Answer from the drawing. Dimensions are ordinates in mm from the lowest x, y and z of the part. Round coordinates to 2 decimals unless told otherwise and drop trailing zeros. Order: outer loops, then holes, each group sorted by start corner. A loop starts at its lowest first (then second) coordinate and runs counter-clockwise, first axis right, second up. Notation, with made-up numbers: (28.25, 81) -> (54.25, 81) arc R31 cw to (54.25, 111) -> close; hole circle Ø5 at (49.5, 19). An arc over 180 degrees is marked (long way). Use a Markdown table: item, result. Add a question column.
1. Section A-A, the plane x = 22 is taken. Give the vertices of the cut face in (y, z), then the cut area to 3 significant figures.
2. The mould has two halves that part along Z. Classify the marked faces 1, 2 and 3: +Z half, -Z half, draft (parallel to the pull), parting line (faces both ways), or undercut.
3. Section B-B, the plane z = 26 is taken. Give the vertices of the cut face in (x, y).
4. Section C-C, the plane y = 37 is taken. Give the vertices of the cut face in (x, z) (1 decimal).
5. Consider L1, parallel to X at y = 6.5, z = 20.5; L2, parallel to Z at x = 31, y = 12.5 (1 decimal); L3, parallel to Z at x = 26, y = 30. Determine where each line is inside the solid, lowest interval first. Write a range as [from, to].
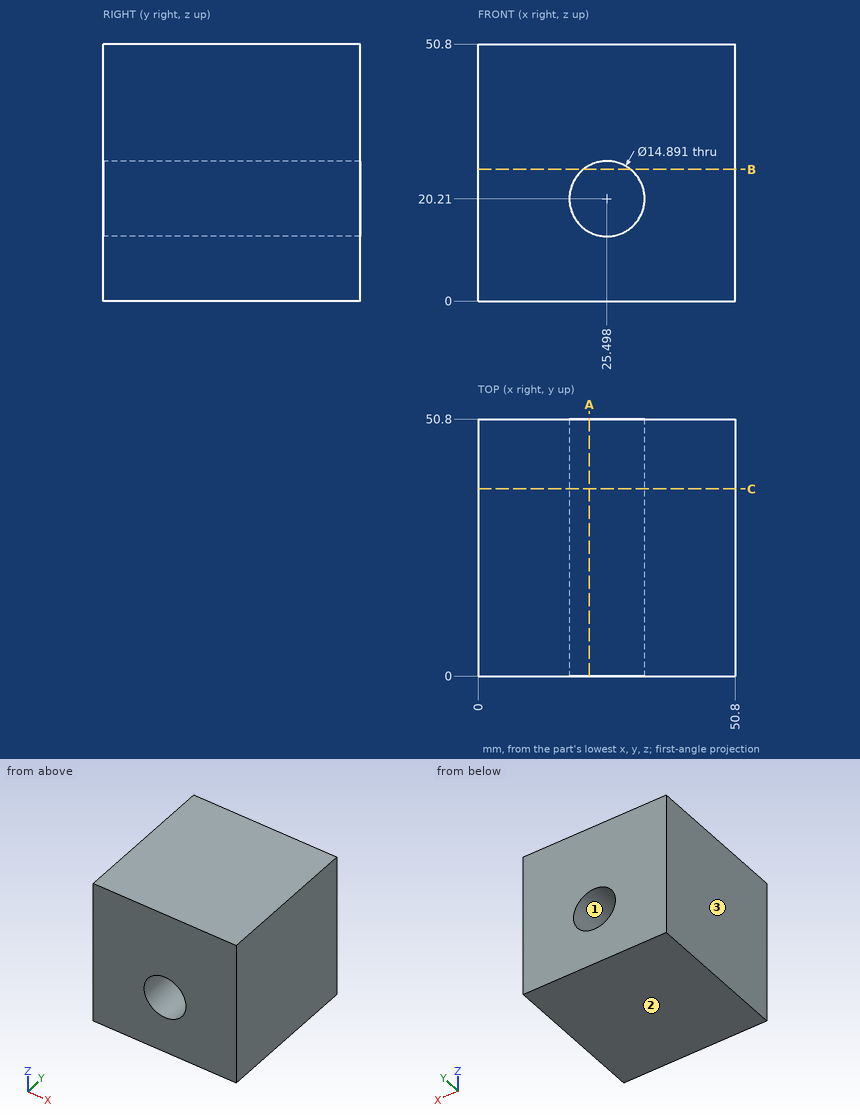
Verdict:
| question | item | result |
|---|---|---|
| 1 | outline | (0, 0) -> (50.8, 0) -> (50.8, 13.64) -> (0, 13.64) -> close; (0, 26.78) -> (50.8, 26.78) -> (50.8, 50.8) -> (0, 50.8) -> close |
| 1 | area | 1,910 mm2 |
| 2 | face 1 | undercut |
| 2 | face 2 | -Z half |
| 2 | face 3 | draft |
| 3 | outline | (0, 0) -> (20.82, 0) -> (20.82, 50.8) -> (0, 50.8) -> close; (30.18, 0) -> (50.8, 0) -> (50.8, 50.8) -> (30.18, 50.8) -> close |
| 4 | outline | (0, 0) -> (50.8, 0) -> (50.8, 50.8) -> (0, 50.8) -> close; hole circle Ø14.9 at (25.5, 20.2) |
| 5 | L1 | x = [0, 18.06], [32.94, 50.8] |
| 5 | L2 | z = [0, 15.2], [25.2, 50.8] |
| 5 | L3 | z = [0, 12.78], [27.64, 50.8] |
